Autodesk Inventor part; units mm, degrees
ref_plane "YZ Plane" through (0, 0, 0) normal (1, 0, 0) x (0, 1, 0)
ref_plane "XZ Plane" through (0, 0, 0) normal (0, 1, 0) x (-1, 0, 0)
ref_plane "XY Plane" through (0, 0, 0) normal (0, 0, 1) x (1, 0, 0)
sketch "Sketch1" plane through (0, 0, 0) normal (0, 1, 0) x (-1, 0, 0)
  circle A0 centre (12.2927, 22.2918) radius 4
  circle A1 centre (12.2927, 22.2918) radius 7.5
  point P0 (0, 0)
  dimension "d0" = 8
  dimension "d1" = 15
extrude "Extrusion1" add sketch "Sketch1" along normal blind 24
chamfer "Chamfer1" distance 1 distance2 0.5 1 edges at (-8.2927, 24, 22.2918) measured on face at (-18.5146, 24, 21.3744)
fillet "Fillet2" radius 1 1 edges at (-4.7927, 24, 22.2918)
fillet "Fillet3" radius 1 1 edges at (-7.2927, 24, 22.2918)
chamfer "Chamfer2" distance 1 distance2 0.5 1 edges at (-8.2927, 0, 22.2918) measured on face at (-16.2409, 15.6667, 21.6501)
fillet "Fillet4" radius 1 1 edges at (-7.7927, 0, 22.2918)
fillet "Fillet5" radius 1 1 edges at (-4.7927, 0, 22.2918)
Source: CAD feature listing. Evaluate the final solid. Frame: model axes, mm. Coordinates: 2 decimals unless noted, no trailing zeros. Order: outer loops, then holes, each group sorted by start corner. A loop starts at its lowest first (then second) coordinate and runs counter-clockwise, first axis right, second up. Notation, with made-up numbers: M 88.5,79 L 114.5,79 A5 ccw 114.5,87 Z; hole C 64.25,43 d11. An arc over 180 degrees is marked long. Write each question's results on one line, items separated by ' | '. Start each with the question number.
Item 1: First-contact query: pin 1 Ø6 at (x, y) = (-16, 14) entering from +Z; pin 2 Ø6.5 at (x, z) = (-12.29, 22.29) entering from +Y; pin 3 Ø5 at (x, z) = (-13, 24) entering from +Y; pin 4 Ø4 at (y, z) = (19.5, 17.5) entering from +X. Flat tips, straight axial feed; report the tip coordinate or a pass-through.
Item 2: Draft query along X for faces 1 (the face through (-6.765, 11.846, 17.223)), 2 (the face through (-9.345, 12.092, 19.588)), 3 (the face through (-17, 0, 19)). Return one class per face: pulls with the +X half, pulls with the -X half, needs draft (parallel to the pull), parting line crosses it, or undercut.
Item 3: Cut plane A-A (y = 10.5). Return loops of the section in (x, z).
Item 4: Line query: probe 1 along Z at (x, y) = (-12.5, 8.25); probe 2 along X at (y, z) = (1, 22.25); probe 3 along Z at (x, y) = (-13.5, 1). Output: solid intervals per line, ascending.
Checked values:
1) pin 1: stops at z = 29.76 | pin 2: passes through | pin 3: stops at y = 23.67 | pin 4: stops at x = -5.33
2) face 1: parting line crosses it | face 2: undercut | face 3: needs draft
3) outline: C -12.29,22.29 d15; hole C -12.29,22.29 d8
4) probe 1: z = 14.79 to 18.3, 26.29 to 29.79 | probe 2: x = -19.79 to -16.29, -8.29 to -4.79 | probe 3: z = 14.89 to 18.48, 26.11 to 29.69
